Read the model definition and answer for the solid it produces. Units are mm, in the model's axes. A direction names the side the tool comes from. Give positions to 0.01 mm unless a question says otherwise; leave off trailing zeros. Order: outer loops, then holes, each group sorted by start corner. A loop starts at its lowest first (then second) coordinate and runs counter-clockwise, first axis right, second up.
Autodesk Inventor part; units mm, degrees
ref_plane "YZ Plane" through (0, 0, 0) normal (1, 0, 0) x (0, 1, 0)
ref_plane "XZ Plane" through (0, 0, 0) normal (0, 1, 0) x (-1, 0, 0)
ref_plane "XY Plane" through (0, 0, 0) normal (0, 0, 1) x (1, 0, 0)
sketch "Esboço2" plane through (0, 0, 0) normal (0, 1, 0) x (-1, 0, 0)
  circle A0 centre (0, 0) radius 1.5
  line L0 (2.7, -1.5588) -> (0, -3.1177)
  line L1 (0, -3.1177) -> (-2.7, -1.5588)
  line L2 (-2.7, -1.5588) -> (-2.7, 1.5588)
  line L3 (-2.7, 1.5588) -> (0, 3.1177)
  line L4 (0, 3.1177) -> (2.7, 1.5588)
  line L5 (2.7, 1.5588) -> (2.7, -1.5588)
extrude "Extrusão1" add sketch "Esboço2" along normal blind 15
thread "Rosca1"
chamfer "Chanfro1" distance 0.3 angle 45 2 edges at (1.5, 15, 0) (1.5, 0, 0)
sketch "Esboço3" plane through (0, 0, 0) normal (0, 0, 1) x (1, 0, 0)
  line L0 (0, -0.48) -> (0, 2.88)
  line L1 (2.4, 0) -> (4.5158, 0.9866)
  line L2 (2.4, 0) -> (4.5158, 0.9866)
  line L3 (4.5158, 0.9866) -> (4.5158, 0)
  line L4 (4.5158, 0.9866) -> (2.4, 0)
  line L5 (2.4, 0) -> (4.5158, 0)
  line L6 (2.7, 0) -> (0, 0)
  line L7 (2.4, 2.4) -> (2.4, 15.0122)
  line L8 (4.5158, 15.0122) -> (2.4, 15.0122)
  line L9 (4.5158, 15.0122) -> (4.5158, 14.0252)
  line L10 (4.5158, 14.0252) -> (2.4, 15.0122)
  dimension "d19" = 0.987
revolve "Revolução3" cut sketch "Esboço3" angle 360 about axis through (0, -10, 0) along (0, 1, 0)
sketch "Esboço4" plane through (0, 15, 0) normal (0, 1, 0) x (1, 0, 0)
  circle A0 centre (0, 0) radius 2.4262
extrude "Extrusão2" add sketch "Esboço4" against normal blind 1.5
sketch "Esboço5" plane through (0, 15, 0) normal (0, 1, 0) x (1, 0, 0)
  circle A0 centre (0, 0) radius 1.5
  dimension "d23" = 3
extrude "Extrusão3" add sketch "Esboço5" along normal blind 4
thread "Rosca2"
properties part number "espaçador 15mm m3" material "Aço galvanizado"
1) Consider L1, parallel to X at y = 5, z = 0; L2, parallel to Y at x = 1.8, z = 0.5; L3, parallel to Z at x = 0.2, y = 9.5. Determine where each line is inside the solid, lowest interval first.
Final values:
L1: x = -2.7 to -1.5, 1.5 to 2.7
L2: y = 0 to 15
L3: z = -3 to -1.49, 1.49 to 3
2) Given pin 1 (1.5 mm diameter, centred on x = -0.5, z = 2, fed in from -Y); pin 2 (1 mm diameter, centred on x = -1.5, y = 9, fed in from -Z); pin 3 (2.5 mm diameter, centred on x = 0, z = 0, fed in from -Y); pin 4 (1 mm diameter, centred on x = -0.5, y = 15, fed in from -Z), each flat-ended and moving along its own axis, determine where each tip first touches the part or whether it passes through.
Final values:
pin 1: stops at y = 0
pin 2: stops at z = -2.54
pin 3: stops at y = 13.5
pin 4: stops at z = -3.06
3) The part is cut by section C-C on y = 17.75. Determine the outline of the cut face in (x, z).
Final values:
outline: circle Ø3 at (0, 0)
4) The part is cut by section A-A on y = 12.5. Determine the outline of the cut face in (x, z), and give its area (3 significant figures).
Final values:
outline: (-2.7, -1.56) - (0, -3.12) - (2.7, -1.56) - (2.7, 1.56) - (0, 3.12) - (-2.7, 1.56) - close; hole circle Ø3 at (0, 0)
area: 18.2 mm2
5) For a pull along X with two mould halves and no side action, classify faces 4 (the face through (0, 19, 0)), 5 (the face through (1.369, 7.403, 2.327)), 6 (the face through (1.5, 6.81, -0.07)) as released by +X, released by -X, zero draft, split by the parting line, or undercut.
Final values:
face 4: zero draft
face 5: released by +X
face 6: undercut
6) A tool of negligible diameter and unlimited length cuts with its end or side. For faces 1 (the face through (1.33, 7.4, -2.35)), 2 (the face through (0, 15, 2)), 3 (the face through (0, 13.5, 0)), from which of +Z, -Z, +X, -X, +Y, -Y can it reach the whole face along a straight path? Write none if from no direction.
Final values:
face 1: -Z, +X, +Y, -Y
face 2: +Y
face 3: -Y
